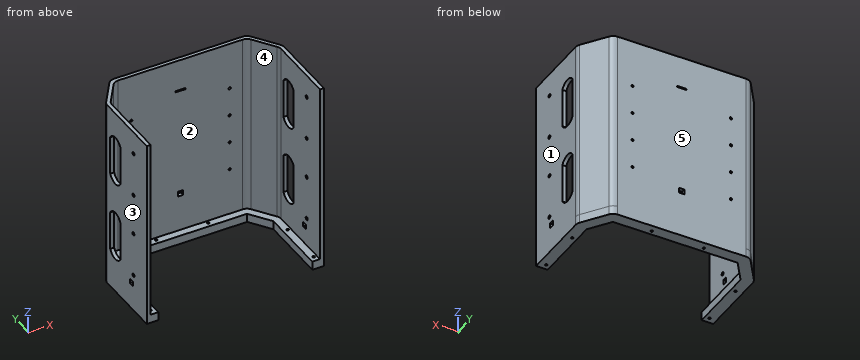
```python
from build123d import *

# Parameters (mm, degrees)
SALIENTE_EXTRUIR1_DEPTH     = 700
REDONDEO1_R                 = 30
CORTAR_EXTRUIR7_DEPTH       = 1052.205028246
ESCALA1_SCALE               = 0.6
ESCALA2_SCALE               = 0.75
CROQUIS17_R                 = 2
CORTAR_EXTRUIR8_DEPTH       = 10
CROQUIS18_R                 = 3
CORTAR_EXTRUIR9_DEPTH       = 677.637223959
CROQUIS19_W                 = 17
CROQUIS19_H                 = 2.2
CORTAR_EXTRUIR10_DEPTH      = 730.049540368
CROQUIS21_W                 = 9
CROQUIS21_H                 = 9
CORTAR_EXTRUIR11_DEPTH      = 674.611531483
CORTAR_EXTRUIR11_DEPTH_BACK = 674.611531483
CROQUIS22_W                 = 9
CROQUIS22_H                 = 9
CORTAR_EXTRUIR12_DEPTH      = 728.451307564
SALIENTE_EXTRUIR3_DEPTH     = 15
CROQUIS26_R                 = 2
CORTAR_EXTRUIR13_DEPTH      = 678.196192286


with BuildPart() as part:
    # Croquis1 → Saliente-Extruir1 (new body)
    with BuildSketch(Plane.XY):
        Polygon((0, 0), (0, 280), (77.5, 390.681470523), (602.5, 390.681470523), (680, 280), (680, 0), (665, 0), (665, 275.270518167), (594.691494242, 375.681470523), (85.308505758, 375.681470523), (15, 275.270518167), (15, 0), align=None)
    extrude(amount=SALIENTE_EXTRUIR1_DEPTH)

    # Redondeo1
    redondeo1_edges = [part.edges().sort_by_distance(p)[0] for p in [
        (0, 280, 350),
        (77.5, 390.681470523, 350),
        (602.5, 390.681470523, 350),
        (680, 280, 350),
        (665, 275.270518167, 350),
        (594.691494242, 375.681470523, 350),
        (85.308505758, 375.681470523, 350),
        (15, 275.270518167, 350),
    ]]
    fillet(redondeo1_edges, radius=REDONDEO1_R)

    # Croquis16 → Cortar-Extruir7 (cut, through all)
    with BuildSketch(Plane(origin=(680, 0, 0), x_dir=(0, 0, -1), z_dir=(1, 0, 0))):
        with BuildLine():
            Line((-430, 180), (-580, 180))
            ThreePointArc((-580, 180), (-600.635083269, 215), (-580, 250))
            Line((-580, 250), (-430, 250))
            ThreePointArc((-430, 250), (-409.364916731, 215), (-430, 180))
        make_face()
    cortar_extruir7 = extrude(amount=-CORTAR_EXTRUIR7_DEPTH, mode=Mode.SUBTRACT)

    # Simetría1: Cortar-Extruir7 across plane
    add(cortar_extruir7.mirror(Plane.XY.offset(350)), mode=Mode.SUBTRACT)


with BuildPart() as part_1:
    # Escala1: scaled about (340, 274.108807771, 350)
    add(part.part.scale(ESCALA1_SCALE).moved(Location((136, 109.643523108, 140))))


with BuildPart() as part_2:
    # Escala2: scaled about (340, 274.108807771, 350)
    add(part_1.part.scale(ESCALA2_SCALE).moved(Location((85, 68.527201943, 87.5))))

    # Croquis17 → Cortar-Extruir8 (cut)
    with BuildSketch(Plane.XZ.offset(-319.816506009)):
        with Locations(Location((255.002655182, 425, 0), (0, 0, 270))):
            Circle(CROQUIS17_R)
        with Locations(Location((255.002655182, 375, 0), (0, 0, 270))):
            Circle(CROQUIS17_R)
        with Locations(Location((425.002655182, 425, 0), (0, 0, 270))):
            Circle(CROQUIS17_R)
        with Locations(Location((255.002655182, 325, 0), (0, 0, 270))):
            Circle(CROQUIS17_R)
        with Locations(Location((255.002655182, 275, 0), (0, 0, 270))):
            Circle(CROQUIS17_R)
        with Locations(Location((425.002655182, 375, 0), (0, 0, 270))):
            Circle(CROQUIS17_R)
        with Locations(Location((425.002655182, 325, 0), (0, 0, 270))):
            Circle(CROQUIS17_R)
        with Locations(Location((425.002655182, 275, 0), (0, 0, 270))):
            Circle(CROQUIS17_R)
    extrude(amount=-CORTAR_EXTRUIR8_DEPTH, mode=Mode.SUBTRACT)

    # Croquis18 → Cortar-Extruir9 (cut, through all)
    with BuildSketch(Plane(origin=(493, 0, 0), x_dir=(0, 0, -1), z_dir=(1, 0, 0))):
        with Locations(Location((-467.5, 191.759844274, 0), (0, 0, 90))):
            Circle(CROQUIS18_R)
        with Locations(Location((-391, 191.759844274, 0), (0, 0, 90))):
            Circle(CROQUIS18_R)
        with Locations(Location((-319, 191.759844274, 0), (0, 0, 90))):
            Circle(CROQUIS18_R)
        with Locations(Location((-242.5, 191.759844274, 0), (0, 0, 90))):
            Circle(CROQUIS18_R)
    extrude(amount=-CORTAR_EXTRUIR9_DEPTH, mode=Mode.SUBTRACT)

    # Croquis19 → Cortar-Extruir10 (cut, through all)
    with BuildSketch(Plane(origin=(0, 326.566506009, 0), x_dir=(1, 0, 0), z_dir=(0, 1, 0))):
        with Locations((340, -451.4)):
            Rectangle(CROQUIS19_W, CROQUIS19_H)
    extrude(amount=-CORTAR_EXTRUIR10_DEPTH, mode=Mode.SUBTRACT)

    # Croquis21 → Cortar-Extruir11 (cut, two sides)
    with BuildSketch(Plane.ZY.offset(-486.25)) as cortar_extruir11_sk:
        with Locations((225, 198.259844274)):
            Rectangle(CROQUIS21_W, CROQUIS21_H)
    extrude(amount=CORTAR_EXTRUIR11_DEPTH, mode=Mode.SUBTRACT)
    extrude(cortar_extruir11_sk.sketch, amount=-CORTAR_EXTRUIR11_DEPTH_BACK, mode=Mode.SUBTRACT)

    # Croquis22 → Cortar-Extruir12 (cut, through all)
    with BuildSketch(Plane.XZ.offset(-319.816506009)):
        with Locations((340, 260)):
            Rectangle(CROQUIS22_W, CROQUIS22_H)
    extrude(amount=-CORTAR_EXTRUIR12_DEPTH, mode=Mode.SUBTRACT)

    # Croquis24 → Saliente-Extruir3 (add)
    with BuildSketch(Plane(origin=(0, 0, 192.5), x_dir=(-1, 0, 0), z_dir=(0, 0, -1))):
        with BuildLine():
            Line((-187, 272.503310624), (-187, 150.759844274))
            Line((-187, 150.759844274), (-207, 150.759844274))
            Line((-207, 150.759844274), (-207, 270.453868496))
            Line((-207, 270.453868496), (-232.286341011, 306.566506009))
            Line((-232.286341011, 306.566506009), (-447.713658989, 306.566506009))
            Line((-447.713658989, 306.566506009), (-473, 270.453868496))
            Line((-473, 270.453868496), (-473, 150.759844274))
            Line((-473, 150.759844274), (-493, 150.759844274))
            Line((-493, 150.759844274), (-493, 272.503310624))
            ThreePointArc((-493, 272.503310624), (-492.375178835, 276.562838918), (-490.558552598, 280.246592515))
            Line((-490.558552598, 280.246592515), (-462.155897415, 320.8097879))
            ThreePointArc((-462.155897415, 320.8097879), (-457.330951096, 325.041152257), (-451.097344818, 326.566506009))
            Line((-451.097344818, 326.566506009), (-228.902655182, 326.566506009))
            ThreePointArc((-228.902655182, 326.566506009), (-222.669048904, 325.041152257), (-217.844102585, 320.8097879))
            Line((-217.844102585, 320.8097879), (-189.441447402, 280.246592515))
            ThreePointArc((-189.441447402, 280.246592515), (-187.624821165, 276.562838918), (-187, 272.503310624))
        make_face()
    extrude(amount=SALIENTE_EXTRUIR3_DEPTH)

    # Croquis26 → Cortar-Extruir13 (cut, through all)
    with BuildSketch(Plane(origin=(0, 0, 177.5), x_dir=(-1, 0, 0), z_dir=(0, 0, -1))):
        with Locations((-385, 314.566506009)):
            Circle(CROQUIS26_R)
        with Locations((-295, 314.566506009)):
            Circle(CROQUIS26_R)
        with Locations((-481, 160.759844274)):
            Circle(CROQUIS26_R)
        with Locations((-199, 160.759844274)):
            Circle(CROQUIS26_R)
        with Locations((-199, 240.759844274)):
            Circle(CROQUIS26_R)
        with Locations((-481, 240.759844274)):
            Circle(CROQUIS26_R)
    extrude(amount=-CORTAR_EXTRUIR13_DEPTH, mode=Mode.SUBTRACT)


solid = part_2.part
```
Here's how the part is built. I have some questions about the finished solid (model axes, mm). Face numbers are marked on the shaded views. A direction names the side the tool comes from. Give positions to 0.01 mm unless a question says otherwise; leave off trailing zeros. Loops run counter-clockwise (first coordinate to the right, second up) from the corner with the lowest first, then second, coordinate; pieces in that order, holes last. Notation, with made-up numbers: M 50,-33 L 55,-33 A11 cw 55,-18 Z; hole C 47.5,64.5 d11. An arc over 180 degrees is marked long. Put each result on its own line as item: value. Start each with the question number.
(1) I want a section at D-D on y = 256.5. Please give me the cut outline in (x, z).
(2) I want a section at B-B on z = 211. Please give me the cut outline in (x, y).
(3) I want a section at A-A on y = 213.5. Please give me the cut outline in (x, z).
(4) If we mould it in two halves opening along X, with no side actions, what happens to the marked faces 3, 4 and 5? For each: +X half, -X half, draft (parallel to the pull), parting line (faces both ways), or undercut.
(5) Will these pins go through, and if not, where does the flat tip stop? pin 1 Ø2 at (x, z) = (488.5, 274.5) entering from +Y; pin 2 Ø4.5 at (x, y) = (481, 240.76) entering from +Z; pin 3 Ø2 at (y, z) = (324.5, 262) entering from +X.
(6) I want a section at C-C on x = 443. Please give me the cut outline in (y, z).
(7) For the marked faces 1 and 2, which set-ups out of +Z, -Z, +X, -X, +Y, -Y let a thin tool reach every point of the face, with its end or its side?
(8) I need wall thicknesses on line 1 along X through (y, z) = (221, 373); line 2 along Y through (x, z) = (189, 391); line 3 along X through (y, z) = (324, 325). Which ranges of each line are inside material? Lowest first, please. Write a range as [from, to].
Answer block:
1. outline: M 187,177.5 L 207,177.5 L 207,192.5 L 193.75,192.5 L 193.75,239.62 L 187,239.62 Z; M 187,320.88 L 193.75,320.88 L 193.75,379.12 L 187,379.12 Z; M 187,460.38 L 193.75,460.38 L 193.75,507.5 L 187,507.5 Z; M 473,177.5 L 493,177.5 L 493,239.62 L 486.25,239.62 L 486.25,192.5 L 473,192.5 Z; M 486.25,320.88 L 493,320.88 L 493,379.12 L 486.25,379.12 Z; M 486.25,460.38 L 493,460.38 L 493,507.5 L 486.25,507.5 Z
2. outline: M 187,150.76 L 193.75,150.76 L 193.75,270.38 A13.5 cw 196.19,278.12 L 221.36,314.06 A13.5 cw 232.42,319.82 L 447.58,319.82 A13.5 cw 458.64,314.06 L 483.81,278.12 A13.5 cw 486.25,270.38 L 486.25,150.76 L 493,150.76 L 493,272.5 A13.5 ccw 490.56,280.25 L 462.16,320.81 A13.5 ccw 451.1,326.57 L 228.9,326.57 A13.5 ccw 217.84,320.81 L 189.44,280.25 A13.5 ccw 187,272.5 Z
3. outline: M 187,177.5 L 207,177.5 L 207,192.5 L 193.75,192.5 L 193.75,507.5 L 187,507.5 Z; M 473,177.5 L 493,177.5 L 493,507.5 L 486.25,507.5 L 486.25,192.5 L 473,192.5 Z
4. face 3: -X half
4. face 4: undercut
4. face 5: draft
5. pin 1: y = 284.61
5. pin 2: z = 192.5
5. pin 3: x = 459.66
6. outline: M 306.57,177.5 L 326.57,177.5 L 326.57,507.5 L 319.82,507.5 L 319.82,192.5 L 306.57,192.5 Z
7. face 1: +Z, -Z, +X, +Y, -Y
7. face 2: +Z, -Y
8. line 1: [187, 193.75], [486.25, 493]
8. line 2: [150.76, 188.76], [194.76, 231.76], [263.26, 279.57]
8. line 3: [220.98, 253], [257, 423], [427, 459.02]
